Check sheet for the drawn part. Datum: minimum x, y, z corner. Units: mm. Round coordinates to 2 decimals unless told otherwise and drop trailing zeros. Write each loop counter-clockwise with the first axis right and the second up, starting at its lowest first coordinate (ties: lowest second). Pieces come first, ordered by that corner, then holes. Notation, with made-up numbers: (81.25, 21) - (112.25, 21) arc R22 ccw to (112.25, 35) - close; hole circle Ø10 at (35, 65). An arc over 180 degrees is marked (long way). Answer as a JSON object with one key per item and string values.
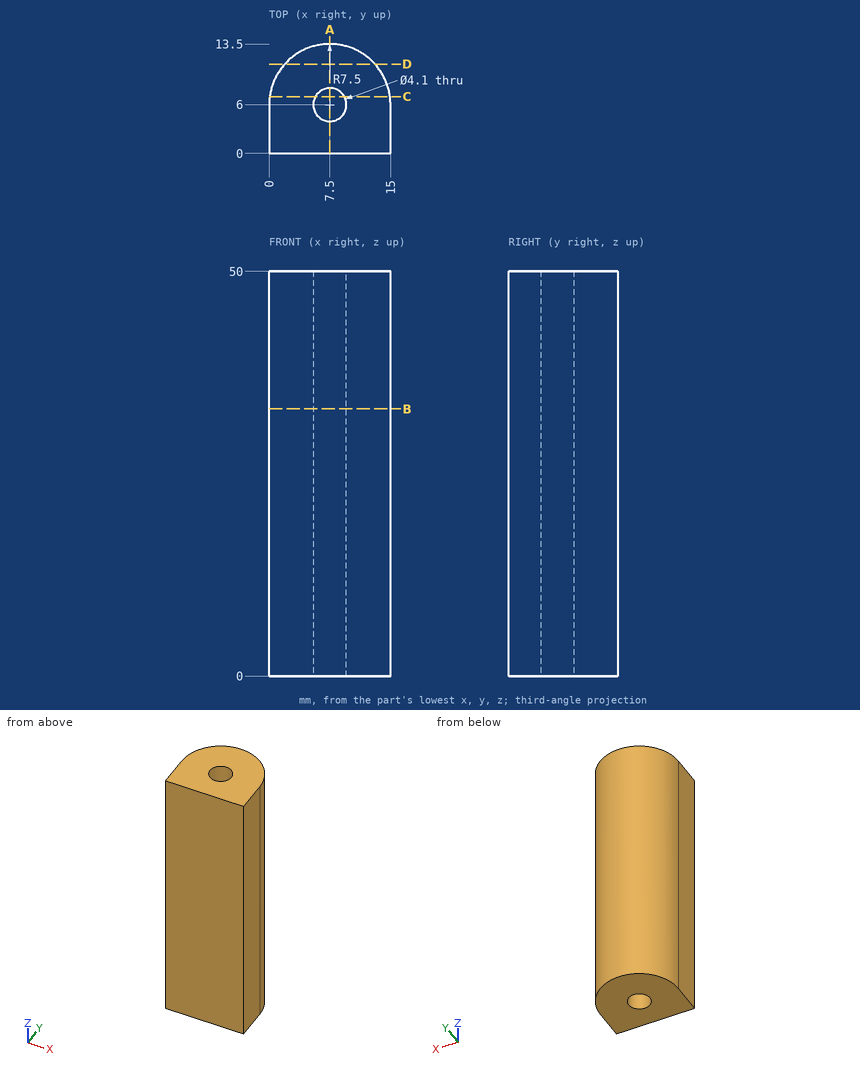
1. Material ranges on probe 1 along Y at (x, z) = (7.5, 28); probe 2 along Y at (x, z) = (6.75, 14); probe 3 along X at (y, z) = (4.5, 4), recorded low to high. Write a range as from..to.
Completed:
{"probe 1": "y = 0..3.95, 8.05..13.5", "probe 2": "y = 0..4.09, 7.91..13.46", "probe 3": "x = 0..6.1, 8.9..15"}
2. Go/stop test with flat-tipped pins: pin 1 (6.5 mm diameter, centred on x = 7.5, y = 6, fed in from -Z); pin 2 (1 mm diameter, centred on y = 9.5, z = 11.5, fed in from -X). Record where each tip stops, or that it passes through.
Completed:
{"pin 1": "stops at z = 0", "pin 2": "stops at x = 0.63"}
3. Cross-section at C-C (y = 7). Record the boundary of the cut face in (x, z), plus the area to 3 significant figures.
Completed:
{"outline": "(0.07, 0) - (5.71, 0) - (5.71, 50) - (0.07, 50) - close; (9.29, 0) - (14.93, 0) - (14.93, 50) - (9.29, 50) - close", "area": "564 mm^2"}
4. Cross-section at A-A (x = 7.5). Record the boundary of the cut face in (y, z), plus the area to 3 significant figures.
Completed:
{"outline": "(0, 0) - (3.95, 0) - (3.95, 50) - (0, 50) - close; (8.05, 0) - (13.5, 0) - (13.5, 50) - (8.05, 50) - close", "area": "470 mm^2"}
5. Cross-section at D-D (y = 11). Record the boundary of the cut face in (x, z), plus the area to 3 significant figures.
Completed:
{"outline": "(1.91, 0) - (13.09, 0) - (13.09, 50) - (1.91, 50) - close", "area": "559 mm^2"}
6. Cross-section at B-B (z = 33). Record the boundary of the cut face in (x, y), plus the area to 3 significant figures.
Completed:
{"outline": "(0, 0) - (15, 0) - (15, 6) arc R7.5 ccw to (0, 6) - close; hole circle Ø4.1 at (7.5, 6)", "area": "165 mm^2"}
